Could you check a few things on this model? Use its own coordinates, in mm. Give positions to 0.01 mm unless a question says otherwise; leave off trailing zeros. Loops run counter-clockwise (first coordinate to the right, second up) from the corner with the lowest first, then second, coordinate; pieces in that order, holes last. Notation, with made-up numbers: (18, -24) - (56, -24) arc R24 ccw to (56, -9) - close; hole circle Ø5 at (5.5, -12.5). An arc over 180 degrees is marked (long way). Write each question's results on one line, items separated by ' | '. Start each with the question number.
(1) Suppose I cut it at B-B (x = 0). Please give me the cut outline in (y, z), and give its area (3 significant figures).
(2) Suppose I cut it at A-A (z = -13). Please give me the cut outline in (x, y).
(3) If we mould it in two halves opening along X, with no side actions, what happens to faces 1 (the face through (-32.198, 10.097, 2.028)), 2 (the face through (1, 20, 0)), 3 (the face through (-41.5, 20, -6)), 4 (the face through (39, 2, -14))? For each: released by +X, released by -X, zero draft, split by the parting line, or undercut.
(4) For pin 1 (7 mm diameter, centred on x = 30, y = 10, fed in from +Z); pin 2 (3.5 mm diameter, centred on x = 0, y = 10, fed in from -Z); pin 3 (2 mm diameter, centred on x = 14, y = 21.5, fed in from -Z), each with a flat end and sliding along its axis, tell me the tip position at first contact or that it passes through.
(5) Suppose I cut it at D-D (y = 26.5). Please give me the cut outline in (x, z), and give its area (3 significant figures).
(6) I need wall thicknesses on line 1 (Y direction, x = -30, z = 1.7); line 2 (X direction, y = 13.5, z = -11); line 3 (X direction, y = 33, z = 1.5). Which ranges of each line are inside material? Lowest first, please.
(7) Suppose I cut it at C-C (z = -7.75). Please give me the cut outline in (x, y).
from build123d import *

# Parameters (mm, degrees)
BOSS_EXTRUDE1_DEPTH = 40
FILLET1_R           = 5
SKETCH2_R           = 2.2
CUT_EXTRUDE1_DEPTH  = 40
SKETCH3_R           = 2.2
CUT_EXTRUDE2_DEPTH  = 94


with BuildPart() as part:
    # Sketch1 → Boss-Extrude1 (new body)
    with BuildSketch(Plane(origin=(0, 0, 0), x_dir=(1, 0, 0), z_dir=(0, 1, 0))):
        with BuildLine():
            Line((36.5, 0), (-36.5, 0))
            Line((-36.5, 0), (-37.5, 0))
            Line((-37.5, 0), (-37.5, 1))
            Line((-37.5, 1), (-37.5, 15))
            Line((-37.5, 15), (-41.5, 15))
            Line((-41.5, 15), (-41.5, -3))
            ThreePointArc((-41.5, -3), (-41.207106781, -3.707106781), (-40.5, -4))
            Line((-40.5, -4), (40.5, -4))
            ThreePointArc((40.5, -4), (41.207106781, -3.707106781), (41.5, -3))
            Line((41.5, -3), (41.5, 15))
            Line((41.5, 15), (37.5, 15))
            Line((37.5, 15), (37.5, 1))
            Line((37.5, 1), (37.5, 0))
            Line((37.5, 0), (36.5, 0))
        make_face()
    extrude(amount=BOSS_EXTRUDE1_DEPTH)

    # Fillet1
    fillet1_edges = [part.edges().sort_by_distance(p)[0] for p in [
        (39.5, 0, -15),
        (-39.5, 0, -15),
        (39.5, 40, -15),
        (-39.5, 40, -15),
    ]]
    fillet(fillet1_edges, radius=FILLET1_R)

    # Sketch2 → Cut-Extrude1 (cut)
    with BuildSketch(Plane.XY.offset(4)):
        with Locations((-30, 32)):
            Circle(SKETCH2_R)
        with Locations((-15, 32)):
            Circle(SKETCH2_R)
        with Locations((0, 32)):
            Circle(SKETCH2_R)
        with Locations((15, 32)):
            Circle(SKETCH2_R)
        with Locations((30, 32)):
            Circle(SKETCH2_R)
        with Locations((-30, 10)):
            Circle(SKETCH2_R)
        with Locations((-15, 10)):
            Circle(SKETCH2_R)
        with Locations((0, 10)):
            Circle(SKETCH2_R)
        with Locations((15, 10)):
            Circle(SKETCH2_R)
        with Locations((30, 10)):
            Circle(SKETCH2_R)
    extrude(amount=-CUT_EXTRUDE1_DEPTH, mode=Mode.SUBTRACT)

    # Sketch3 → Cut-Extrude2 (cut)
    with BuildSketch(Plane.ZY.offset(41.5)):
        with Locations((-7.5, 30)):
            Circle(SKETCH3_R)
        with Locations((-7.5, 8)):
            Circle(SKETCH3_R)
    extrude(amount=-CUT_EXTRUDE2_DEPTH, mode=Mode.SUBTRACT)


solid = part.part
Output values:
1) outline: (0, 0) - (7.8, 0) - (7.8, 4) - (0, 4) - close; (12.2, 0) - (29.8, 0) - (29.8, 4) - (12.2, 4) - close; (34.2, 0) - (40, 0) - (40, 4) - (34.2, 4) - close | area: 125 mm2
2) outline: (-41.5, 1) - (-37.5, 1) - (-37.5, 39) - (-41.5, 39) - close; (37.5, 1) - (41.5, 1) - (41.5, 39) - (37.5, 39) - close
3) face 1: undercut | face 2: undercut | face 3: released by -X | face 4: zero draft
4) pin 1: z = 4 | pin 2: through | pin 3: z = 0
5) outline: (-41.5, -15) - (-37.5, -15) - (-37.5, 0) - (37.5, 0) - (37.5, -15) - (41.5, -15) - (41.5, 3) arc R1 ccw to (40.5, 4) - (-40.5, 4) arc R1 ccw to (-41.5, 3) - close | area: 452 mm2
6) line 1: 0 to 7.8, 12.2 to 29.8, 34.2 to 40 | line 2: -41.5 to -37.5, 37.5 to 41.5 | line 3: -41.5 to -31.96, -28.04 to -16.96, -13.04 to -1.96, 1.96 to 13.04, 16.96 to 28.04, 31.96 to 41.5
7) outline: (-41.5, 0) - (-37.5, 0) - (-37.5, 5.81) - (-41.5, 5.81) - close; (-41.5, 10.19) - (-37.5, 10.19) - (-37.5, 27.81) - (-41.5, 27.81) - close; (-41.5, 32.19) - (-37.5, 32.19) - (-37.5, 40) - (-41.5, 40) - close; (37.5, 0) - (41.5, 0) - (41.5, 5.81) - (37.5, 5.81) - close; (37.5, 10.19) - (41.5, 10.19) - (41.5, 27.81) - (37.5, 27.81) - close; (37.5, 32.19) - (41.5, 32.19) - (41.5, 40) - (37.5, 40) - close
